Part model, mm, in its own coordinate system. A direction names the side the tool comes from. Coordinates: 2 decimals unless noted, no trailing zeros. Order: outer loops, then holes, each group sorted by start corner. A loop starts at its lowest first (then second) coordinate and runs counter-clockwise, first axis right, second up.
from build123d import *

# Parameters (mm, degrees)
SKETCH1_W           = 25.4
SKETCH1_H           = 0.254
BOSS_EXTRUDE1_DEPTH = 1012.444
SKETCH3_W           = 25.4
SKETCH3_H           = 0.254


with BuildPart() as part:
    # Sketch1 → Boss-Extrude1 (new body)
    with BuildSketch(Plane.XY):
        with Locations((12.7, 0.127)):
            Rectangle(SKETCH1_W, SKETCH1_H)
    extrude(amount=BOSS_EXTRUDE1_DEPTH)

    # Sweep12: sweep along a path in Sketch5
    with BuildLine(Plane(origin=(0, 0, 0), x_dir=(0, 0, -1), z_dir=(1, 0, 0))) as sweep12_path:
        ThreePointArc((-880.897498734, 147.072202414), (-902.023368964, 230.752034475), (-862.54915142, 154.003074639))
        Line((-862.54915142, 154.003074639), (-1025.857747632, 44.913935374))
        ThreePointArc((-1025.857747632, 44.913935374), (-1035.666679092, 17.623395262), (-1012.444, 0.254))
    # Sketch3 → Sweep12 (sweep)
    with BuildSketch(Plane.XY.offset(1012.444)):
        with Locations((12.7, 0.127)):
            Rectangle(SKETCH3_W, SKETCH3_H)
    sweep(path=sweep12_path.line)


solid = part.part
Q1. Cut at D-D on z = 102.5. Write the cut outline in (x, y), and give its area (3 significant figures).
Results list:
outline: (0, 0) - (25.4, 0) - (25.4, 0.25) - (0, 0.25) - close
area: 6.45 mm2
Q2. Cut at B-B on z = 968.5. Write the cut outline in (x, y).
Results list:
outline: (0, 0) - (25.4, 0) - (25.4, 0.25) - (0, 0.25) - close; (0, 83.23) - (25.4, 83.23) - (25.4, 83.53) - (0, 83.53) - close
Q3. Cut at C-C on x = 19.5. Write the cut outline in (y, z).
Results list:
outline: (0, 0) - (0.25, 0) - (0.25, 1012.44) arc R24.38 cw to (44.91, 1025.86) - (154, 862.55) arc R43.43 ccw (long way) to (147.07, 880.9) - (147.32, 880.93) arc R43.18 cw (long way) to (154.21, 862.69) - (45.12, 1026) arc R24.64 ccw to (0, 1012.44) - close
Q4. Wall check: line 1 along Z through (x, y) = (10.5, 186); line 2 along Y through (x, z) = (10.25, 925); line 3 along Y through (x, z) = (4, 368.5). Give the ranges that are in metal, low to high.
Results list:
line 1: z = 843.44 to 843.69, 929.66 to 929.91
line 2: y = 0 to 0.25, 112.29 to 112.59, 169.68 to 170.23, 210.01 to 210.56
line 3: y = 0 to 0.25
Q5. Which spindle directions (+Z, -Z, +X, -X, +Y, -Y) get a long thin tool onto all of the face, cutting with end or side? Do faces 1 (the face through (12.878, 229.859, 903.567)), 2 (the face through (12.878, 98.695, 945.347)). Say none if no direction does.
Results list:
face 1: +X, -X
face 2: -Z, +X, -X
Q6. Cut at A-A on y = 165.5. Write the cut outline in (x, z).
Results list:
outline: (0, 850.89) - (25.4, 850.89) - (25.4, 851.2) - (0, 851.2) - close; (0, 922.15) - (25.4, 922.15) - (25.4, 922.46) - (0, 922.46) - close
Q7. Pin check, flat tips, straight feed: pin 1 Ø8 at (x, z) = (13.5, 326) entering from +Y; pin 2 Ø12 at (x, y) = (22.5, 53) entering from -Z; pin 3 Ø6 at (x, z) = (22.5, 850) entering from +Y; pin 4 Ø12 at (x, y) = (11.5, 28.5) entering from +Z. Stop position of each tip, or through.
Results list:
pin 1: stops at y = 0.25
pin 2: stops at z = 1004.77
pin 3: stops at y = 217.55
pin 4: stops at z = 1036.95
Q8. Mould opens along Y. For faces 3 (the face through (12.88, 17.97, 1036.03)), 4 (the face through (13, 0, 499)), 5 (the face through (12.52, 230.09, 903.67)) say: pulls with the +Y half, pulls with the -Y half, needs draft (parallel to the pull), parting line crosses it, or undercut.
Results list:
face 3: parting line crosses it
face 4: pulls with the -Y half
face 5: undercut
